Autodesk Inventor part; units mm, degrees
ref_plane "YZ Plane" through (0, 0, 0) normal (1, 0, 0) x (0, 1, 0)
ref_plane "XZ Plane" through (0, 0, 0) normal (0, 1, 0) x (-1, 0, 0)
ref_plane "XY Plane" through (0, 0, 0) normal (0, 0, 1) x (1, 0, 0)
sketch "Sketch19" plane through (0, 0, 0) normal (0, 1, 0) x (-1, 0, 0)
  arc A0 (-13.4483, -63.5936) -> (-13.4483, 63.5936) centre (0, 0) ccw
  line L0 (-73, -51) -> (-73, 51)
  line L1 (-73, 51) -> (-13.4483, 63.5936)
  line L2 (-73, -51) -> (-13.4483, -63.5936)
  dimension "d91" = 130
  dimension "d93" = 102
extrude "Extrusion18" add sketch "Sketch19" along normal blind 37
sketch "Sketch20" plane through (0, 37, 0) normal (0, 1, 0) x (1, 0, 0)
  arc A0 (0, 56) -> (0, -56) centre (0, 0) ccw
  line L0 (0, -56) -> (0, -65)
  line L1 (0, 56) -> (0, 65)
  arc A1 (13.4483, 63.5936) -> (13.4483, -63.5936) centre (0, 0) ccw
  line L2 (13.4483, -63.5936) -> (73, -51)
  line L3 (73, -51) -> (73, 51)
  line L4 (73, 51) -> (13.4483, 63.5936)
  dimension "d96" = 112
extrude "Extrusion19" add sketch "Sketch20" along normal blind 65 contours L1 A1 L4 L3 L2 L0 A0
chamfer "Chamfer2" distance 9 angle 45 1 edges at (-56, 37, 0)
sketch "Sketch21" plane through (0, 0, 0) normal (0, -1, 0) x (1, 0, 0)
  circle A0 centre (0, 0) radius 29
  dimension "d102" = 58
extrude "Extrusion20" cut sketch "Sketch21" against normal blind 4
sketch "Sketch22" plane through (0, 4, 0) normal (0, -1, 0) x (1, 0, 0)
  circle A0 centre (0, 0) radius 24
  dimension "d105" = 48
extrude "Extrusion21" cut sketch "Sketch22" against normal blind 19
sketch "Sketch23" plane through (0, 0, 0) normal (0, -1, 0) x (1, 0, 0)
  circle A0 centre (-54, 0) radius 5
  circle A1 centre (54, 0) radius 5
  point P0 (0, 0)
  dimension "d109" = 10
  dimension "d110" = 10
extrude "Extrusion22" cut sketch "Sketch23" against normal blind 12
sketch "Sketch24" plane through (73, 0, 51) normal (1, 0, 0) x (0, 0, -1)
  line L0 (0, 102) -> (102, 102)
  line L1 (102, 0) -> (102, 102)
  line L2 (0, 0) -> (0, 102)
  line L3 (0, 0) -> (102, 0)
  circle A0 centre (51, 51) radius 29
  point P0 (51, 0)
  dimension "d113" = 58
extrude "Extrusion23" cut sketch "Sketch24" against normal blind 5 contours A0
sketch "Sketch25" plane through (68, 51, 0) normal (1, 0, 0) x (0, 0, -1)
  circle A0 centre (0, 0) radius 24
  point P0 (0, -51)
  dimension "d116" = 48
extrude "Extrusion24" cut sketch "Sketch25" against normal blind 4
sketch "Sketch26" plane through (64, 51, 0) normal (1, 0, 0) x (0, 0, -1)
  circle A0 centre (0, 0) radius 13.5
  point P0 (0, -51)
  dimension "d119" = 27
extrude "Extrusion25" cut sketch "Sketch26" against normal blind 38
sketch "Sketch27" plane through (73, 0, 51) normal (1, 0, 0) x (0, 0, -1)
  line L0 (15, 86) -> (87, 14) construction
  line L1 (87, 86) -> (15, 14) construction
  circle A0 centre (15, 86) radius 5
  circle A1 centre (87, 86) radius 5
  circle A2 centre (87, 14) radius 5
  circle A3 centre (15, 14) radius 5
  point P0 (51, 0)
  point P1 (51, 50)
  dimension "d125" = 72
  dimension "d126" = 72
  dimension "d127" = 10
  dimension "d128" = 10
  dimension "d129" = 10
  dimension "d130" = 10
extrude "Extrusion26" cut sketch "Sketch27" against normal blind 16
sketch "Sketch28" plane through (0, 102, 0) normal (0, 1, 0) x (1, 0, 0)
  circle A0 centre (0, 0) radius 22.5
  dimension "d133" = 45
extrude "Extrusion27" add sketch "Sketch28" along normal blind 81
sketch "Sketch29" plane through (0, 183, 0) normal (0, 1, 0) x (1, 0, 0)
  circle A0 centre (0, 0) radius 13.5
  dimension "d136" = 27
extrude "Extrusion28" cut sketch "Sketch29" against normal blind 26
sketch "Sketch30" plane through (0, 157, 0) normal (0, 1, 0) x (1, 0, 0)
  circle A0 centre (0, 0) radius 8.5
  dimension "d139" = 17
extrude "Extrusion29" cut sketch "Sketch30" against normal blind 91
sketch "Sketch31" plane through (0, 0, 0) normal (0, 0, 1) x (1, 0, 0)
  line L0 (22.5, 102) -> (22.5, 183)
  line L1 (22.5, 102) -> (22.5, 106)
  line L2 (22.5, 102) -> (26.5, 102) construction
  circle A0 centre (22.5, 104) radius 2
  line L3 (-92.6, 0) -> (100.6, 0)
  line L4 (0, -36.6) -> (0, 219.6)
  point P0 (0, 0)
  dimension "d142" = 4
  dimension "d143" = 90
revolve "Revolution1" cut sketch "Sketch31" angle 360 about axis through (0, -10, 0) along (0, 1, 0)
sketch "Sketch32" plane through (0, 23, 0) normal (0, -1, 0) x (1, 0, 0)
  circle A0 centre (0, 0) radius 29
  dimension "d146" = 58
extrude "Extrusion30" cut sketch "Sketch32" against normal blind 43
thread "Thread10"
thread "Thread11"
thread "Thread12"
thread "Thread13"
thread "Thread14"
thread "Thread15"
thread "Thread16"
thread "Thread17"
properties part number "00.32.001 \"Housing \"" material "Steel"
For this review, take the finished solid that the model builds, in its own axes (mm). A direction names the side the tool comes from. Round coordinates to 2 decimals unless told otherwise and drop trailing zeros. Loops run counter-clockwise (first coordinate to the right, second up) from the corner with the lowest first, then second, coordinate; pieces in that order, holes last. Notation, with made-up numbers: (54.25, -28.5) - (69.25, -28.5) arc R24 cw to (69.25, -6.5) - close; hole circle Ø3 at (30.25, 10.25). An arc over 180 degrees is marked (long way). Put each result on its own line as item: value. Start each with the question number.
1. Consider section C-C on y = 30. State the section outline as (x, z) points.
2. Mouldability with a two-part tool opening along X and no side actions: class faces 1 (the flat face through (-54, 12, 0)), 2 (the cylindrical face through (65, 14, 41)), 3 (the flat face through (54, 12, 0)), 4 (the flat face through (57, 86, -36)) as +X half, -X half, draft (parallel to the pull), parting line (faces both ways), or undercut.
3. For probe 1 along Y at (x, z) = (68.5, 36); probe 2 along Z at (x, y) = (0, 111); probe 3 along Y at (x, z) = (62, 31.5), list the stretches that pass through material, from the lowest coordinate up. Write a range as [from, to].
4. For faces 5 (the cylindrical face through (-28.97, 44.2, 1.28)), 6 (the flat face through (0, 69, 60)), 7 (the cylindrical face through (10.382, 143.961, -19.961)), 8 (the cylindrical face through (45.266, 55.055, -12.877)), list the 3-axis set-ups (+Z, -Z, +X, -X, +Y, -Y) from which the entire face can be reached by the end or side of a thin tool; tool diameter is ignored.
5. Insertion check: P1, Ø6, axis at x = 44, y = 72.5, coming from the -Z side; P2, Ø1.5, axis at x = -12, z = -19.5, coming from the -Y side; P3, Ø8, axis at y = 36, z = 43, coming from the -X side. Each pin has a flat end and moves straight along its axis. Give the tip position at first contact, or say it passes through.
6. Consider section D-D on y = 168.5. State the section outline as (x, z) points, plus the area to 3 significant figures.
7. Consider section B-B on x = 54. State the section outline as (y, z) points, plus the area to 3 significant figures.
Result sheet:
1. outline: (13.45, -63.59) - (73, -51) - (73, -20) - (68, -20) - (68, -11.62) - (64, -11.62) - (64, 11.62) - (68, 11.62) - (68, 20) - (73, 20) - (73, 51) - (13.45, 63.59) arc R65 ccw (long way) to start; hole circle Ø58 at (0, 0)
2. face 1: undercut
2. face 2: draft
2. face 3: undercut
2. face 4: +X half
3. probe 1: [0, 9], [19, 81], [91, 102]
3. probe 2: [-22.5, -8.5], [8.5, 22.5]
3. probe 3: [0, 11.82], [16.18, 83.82], [88.18, 102]
4. face 5: none
4. face 6: +Z, -X, +Y
4. face 7: +Y
4. face 8: +X
5. P1: z = -57.77
5. P2: y = 66
5. P3: x = -52
6. outline: circle Ø45 at (0, 0); hole circle Ø27 at (0, 0)
6. area: 1,020 mm^2
7. outline: (0, -55.02) - (102, -55.02) - (102, 55.02) - (0, 55.02) - (0, 5) - (12, 5) - (12, -5) - (0, -5) - close; hole circle Ø27 at (51, 0)
7. area: 10,500 mm^2
